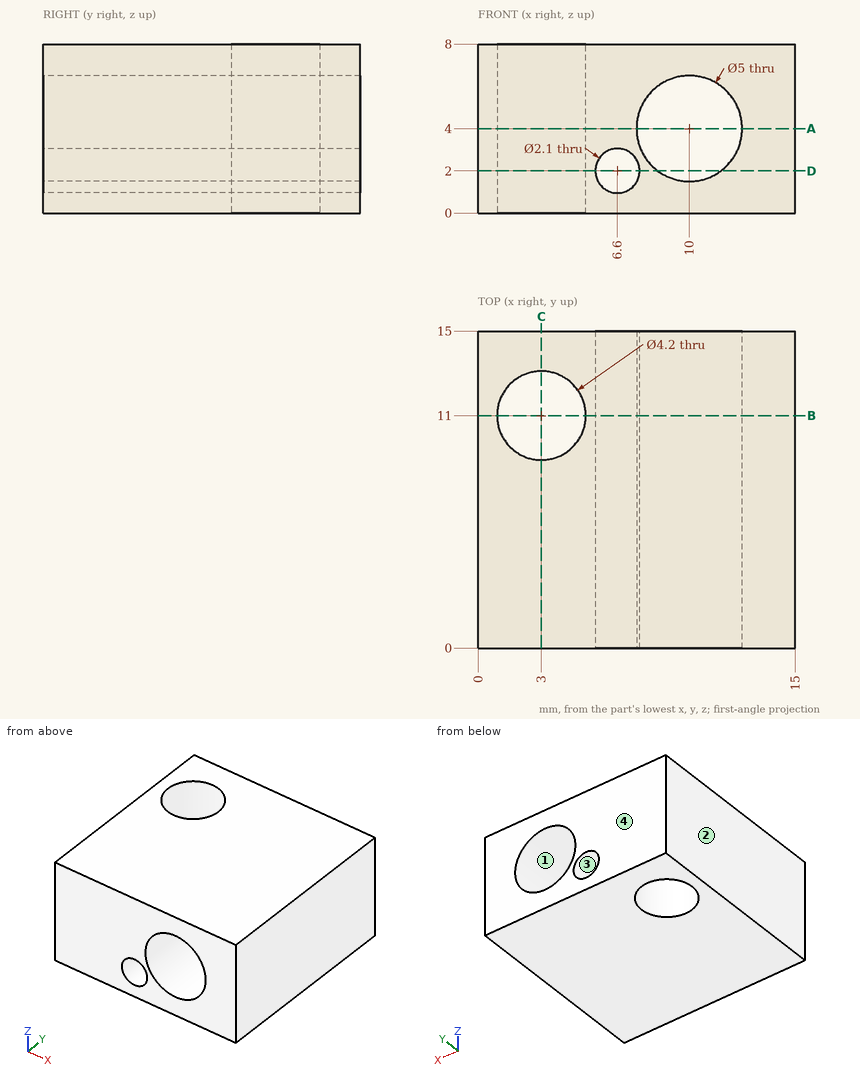
Could you check a few things on this drawing? It's one solid part, dimensions in mm from its lowest x, y, z. Round coordinates to 2 decimals unless told otherwise and drop trailing zeros. Order: outer loops, then holes, each group sorted by start corner. A loop starts at its lowest first (then second) coordinate and runs counter-clockwise, first axis right, second up. Notation, with made-up numbers: (8, -31.75) -> (38, -31.75) arc R14 ccw to (38, -11.75) -> close; hole circle Ø7 at (85, 81). An arc over 180 degrees is marked (long way). One line per question, with ' | ' between items.
Q1. If we section it at B-B on y = 11: Write out the boundary of the cut face in (x, z).
Computed values:
outline: (0, 0) -> (0.9, 0) -> (0.9, 8) -> (0, 8) -> close; (5.1, 0) -> (15, 0) -> (15, 8) -> (5.1, 8) -> close; hole circle Ø2.1 at (6.6, 2); hole circle Ø5 at (10, 4)
Q2. If we section it at A-A on z = 4: Write out the boundary of the cut face in (x, y), plus the area to 3 significant figures.
Computed values:
outline: (0, 0) -> (7.5, 0) -> (7.5, 15) -> (0, 15) -> close; (12.5, 0) -> (15, 0) -> (15, 15) -> (12.5, 15) -> close; hole circle Ø4.2 at (3, 11) | area: 136 mm²
Q3. If we section it at C-C on x = 3: Write out the boundary of the cut face in (y, z), plus the area to 3 significant figures.
Computed values:
outline: (0, 0) -> (8.9, 0) -> (8.9, 8) -> (0, 8) -> close; (13.1, 0) -> (15, 0) -> (15, 8) -> (13.1, 8) -> close | area: 86.4 mm²
Q4. If we section it at D-D on z = 2: Write out the boundary of the cut face in (x, y), plus the area to 3 significant figures.
Computed values:
outline: (0, 0) -> (5.55, 0) -> (5.55, 15) -> (0, 15) -> close; (7.65, 0) -> (8.5, 0) -> (8.5, 15) -> (7.65, 15) -> close; (11.5, 0) -> (15, 0) -> (15, 15) -> (11.5, 15) -> close; hole circle Ø4.2 at (3, 11) | area: 135 mm²
Q5. If I drill on line 1 (X direction, y = 10.5, z = 5.25); line 2 (Z direction, x = 10, y = 10); line 3 (Y direction, x = 3, z = 5.75), over which ranges is the centre line in solid material (lowest first)? Write a range as from..to.
Computed values:
line 1: 0..0.96, 5.04..7.83, 12.17..15 | line 2: 0..1.5, 6.5..8 | line 3: 0..8.9, 13.1..15
Q6. We'd pull the mould along X, two halves only. Please class the marked faces 1, 2, 3 and 4: released by +X, released by -X, zero draft, split by the parting line, or undercut.
Computed values:
face 1: undercut | face 2: released by -X | face 3: undercut | face 4: zero draft
